Model file for the job. Use its own axes, mm. Face numbers are marked on the shaded views. Coordinates: 2 decimals unless noted, no trailing zeros. Order: outer loops, then holes, each group sorted by start corner. A loop starts at its lowest first (then second) coordinate and runs counter-clockwise, first axis right, second up. Notation, with made-up numbers: M -5.75,29 L 10.25,29 A18 cw 10.25,54 Z; hole C -37,45 d8. An arc over 180 degrees is marked long. Return JSON: item names as keys, results as strings.
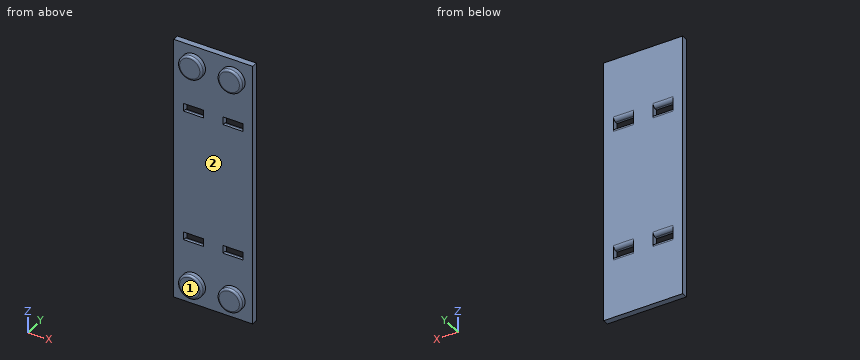
```python
from build123d import *

# Parameters (mm, degrees)
SKETCH1_W           = 40
SKETCH1_H           = 133.5
BOSS_EXTRUDE1_DEPTH = 3
SKETCH2_R           = 6.11
BOSS_EXTRUDE2_DEPTH = 3
CUT_EXTRUDE1_REACH  = 71.94
SKETCH3_W           = 10
SKETCH3_H           = 4
FILLET2_R           = 1.75
FILLET3_R           = 1


with BuildPart() as part:
    # Sketch1 → Boss-Extrude1 (new body)
    with BuildSketch(Plane(origin=(0, 0, 0), x_dir=(1, 0, 0), z_dir=(0, 1, 0))):
        Rectangle(SKETCH1_W, SKETCH1_H)
    extrude(amount=BOSS_EXTRUDE1_DEPTH)

    # Sketch2 → Boss-Extrude2 (add)
    with BuildSketch(Plane.XZ):
        with Locations(Location((10, 56.75, 0), (0, 0, 90))):
            Circle(SKETCH2_R)
        with Locations(Location((-10, 56.75, 0), (0, 0, 90))):
            Circle(SKETCH2_R)
        with Locations(Location((-10, -56.75, 0), (0, 0, 90))):
            Circle(SKETCH2_R)
        with Locations(Location((10, -56.75, 0), (0, 0, 90))):
            Circle(SKETCH2_R)
    extrude(amount=BOSS_EXTRUDE2_DEPTH)

    # Sketch3 → Cut-Extrude1 (cut, up to next)
    with BuildSketch(Plane(origin=(0, 3, 0), x_dir=(1, 0, 0), z_dir=(0, 1, 0)), mode=Mode.PRIVATE) as cut_extrude1_sk1:
        with Locations((10, 33.3125)):
            Rectangle(SKETCH3_W, SKETCH3_H)
    cut_extrude1_tool1 = extrude(cut_extrude1_sk1.sketch, amount=-CUT_EXTRUDE1_REACH, mode=Mode.PRIVATE) & part.part
    # Sketch3 → Cut-Extrude1 (cut, up to next)
    with BuildSketch(Plane(origin=(0, 3, 0), x_dir=(1, 0, 0), z_dir=(0, 1, 0)), mode=Mode.PRIVATE) as cut_extrude1_sk2:
        with Locations((-10, 33.3125)):
            Rectangle(SKETCH3_W, SKETCH3_H)
    cut_extrude1_tool2 = extrude(cut_extrude1_sk2.sketch, amount=-CUT_EXTRUDE1_REACH, mode=Mode.PRIVATE) & part.part
    # Sketch3 → Cut-Extrude1 (cut, up to next)
    with BuildSketch(Plane(origin=(0, 3, 0), x_dir=(1, 0, 0), z_dir=(0, 1, 0)), mode=Mode.PRIVATE) as cut_extrude1_sk3:
        with Locations((-10, -33.3125)):
            Rectangle(SKETCH3_W, SKETCH3_H)
    cut_extrude1_tool3 = extrude(cut_extrude1_sk3.sketch, amount=-CUT_EXTRUDE1_REACH, mode=Mode.PRIVATE) & part.part
    # Sketch3 → Cut-Extrude1 (cut, up to next)
    with BuildSketch(Plane(origin=(0, 3, 0), x_dir=(1, 0, 0), z_dir=(0, 1, 0)), mode=Mode.PRIVATE) as cut_extrude1_sk4:
        with Locations((10, -33.3125)):
            Rectangle(SKETCH3_W, SKETCH3_H)
    cut_extrude1_tool4 = extrude(cut_extrude1_sk4.sketch, amount=-CUT_EXTRUDE1_REACH, mode=Mode.PRIVATE) & part.part
    add(cut_extrude1_tool1.solids().sort_by_distance((10, 3, -33.3125))[0], mode=Mode.SUBTRACT)
    add(cut_extrude1_tool2.solids().sort_by_distance((-10, 3, -33.3125))[0], mode=Mode.SUBTRACT)
    add(cut_extrude1_tool3.solids().sort_by_distance((-10, 3, 33.3125))[0], mode=Mode.SUBTRACT)
    add(cut_extrude1_tool4.solids().sort_by_distance((10, 3, 33.3125))[0], mode=Mode.SUBTRACT)

    # Fillet2
    fillet2_edges = [part.edges().sort_by_distance(p)[0] for p in [
        (10, 3, 35.3125),
        (10, 3, 31.3125),
        (-10, 3, 35.3125),
        (-10, 3, 31.3125),
        (-10, 3, -35.3125),
        (-10, 3, -31.3125),
        (10, 3, -35.3125),
        (10, 3, -31.3125),
    ]]
    fillet(fillet2_edges, radius=FILLET2_R)

    # Fillet3
    fillet3_edges = [part.edges().sort_by_distance(p)[0] for p in [
        (10, -3, -62.86),
        (-10, -3, -62.86),
        (-10, -3, 50.64),
        (10, -3, 50.64),
    ]]
    fillet(fillet3_edges, radius=FILLET3_R)


solid = part.part
```
Item 1: Pull direction Z, two halves, no side cores. Call the marked faces 1 and 2: +Z half, -Z half, draft (parallel to the pull), parting line (faces both ways), or undercut.
Check result:
{"face 1": "draft", "face 2": "undercut"}
Item 2: Saw through at D-D (x = -8.5). Count the separate pieces of the cut face and the enclosed holes in it, and give its area (3 significant figures).
Check result:
{"separate pieces": "3", "enclosed holes": "0", "area": "444 mm2"}
Item 3: Saw through at A-A (x = 10). Write the cut outline in (y, z).
Check result:
{"outline": "M -3,-61.86 A1 ccw -2,-62.86 L 0,-62.86 L 0,-66.75 L 3,-66.75 L 3,-37.06 A1.75 ccw 1.25,-35.31 L 0,-35.31 L 0,-50.64 L -2,-50.64 A1 ccw -3,-51.64 Z; M -3,51.64 A1 ccw -2,50.64 L 0,50.64 L 0,35.31 L 1.25,35.31 A1.75 ccw 3,37.06 L 3,66.75 L 0,66.75 L 0,62.86 L -2,62.86 A1 ccw -3,61.86 Z; M 0,-31.31 L 1.25,-31.31 A1.75 ccw 3,-29.56 L 3,29.56 A1.75 ccw 1.25,31.31 L 0,31.31 Z"}
Item 4: Saw through at B-B (z = 56.75). Write the cut outline in (x, y).
Check result:
{"outline": "M -20,0 L -16.11,0 L -16.11,-2 A1 ccw -15.11,-3 L -4.89,-3 A1 ccw -3.89,-2 L -3.89,0 L 3.89,0 L 3.89,-2 A1 ccw 4.89,-3 L 15.11,-3 A1 ccw 16.11,-2 L 16.11,0 L 20,0 L 20,3 L -20,3 Z"}
Item 5: Wall check: line 1 (X direction, y = 0.95, z = -35); line 2 (Y direction, x = 9, z = 3); line 3 (Z direction, x = -11, y = 2.15). Give the ranges that are in metal, low to high.
Check result:
{"line 1": "x = -20 to -15, -5 to 5, 15 to 20", "line 2": "y = 0 to 3", "line 3": "z = -66.75 to -35.56, -31.06 to 31.06, 35.56 to 66.75"}
Item 6: Saw through at C-C (z = 1). Write the cut outline in (x, y), and give its area (3 significant figures).
Check result:
{"outline": "M -20,0 L 20,0 L 20,3 L -20,3 Z", "area": "120 mm2"}
Item 7: Drop a flat-ended pin along its axis: pin 1 Ø6 at (x, z) = (-7.5, -10) entering from -Y. Give the stop position or say it passes through.
Check result:
{"pin 1": "stops at y = 0"}
